CAD build for the part. Positions are in the model's coordinates, mm. A direction names the side the tool comes from. Give positions to 0.01 mm unless a question says otherwise; leave off trailing zeros. Order: outer loops, then holes, each group sorted by start corner. A loop starts at its lowest first (then second) coordinate and runs counter-clockwise, first axis right, second up. Notation, with made-up numbers: (-5, 59.25) -> (12, 59.25) arc R17 cw to (12, 91.25) -> close; hole circle Ø4 at (11, 73.25). An arc over 180 degrees is marked (long way). Answer as CSV lines item,"result".
```python
from build123d import *

# Parameters (mm, degrees)
SKETCH_2_OUTSIDE_W  = 26.11
SKETCH_2_OUTSIDE_H  = 26.11
CUT_EXTRUDE_1_DEPTH = 45.3


with BuildPart() as part:
    # Эскиз1 → Повернуть1 (revolve)
    with BuildSketch(Plane.XY, mode=Mode.PRIVATE) as revolve_1_sk:
        Polygon((-5.3, 0), (-5.3, 6.175), (-5.052146997, 7.1), (0, 7.1), (0, 4), (39.2, 4), (40, 3.2), (40, 0), align=None)
    revolve(revolve_1_sk.sketch.rotate(Axis((-1000, 0, 0), (1, 0, 0)), 90), axis=Axis((-1000, 0, 0), (1, 0, 0)))

    # Эскиз2 outside → Вырез-Вытянуть1 (cut)
    with BuildSketch(Plane.ZY.offset(5.3)):
        Rectangle(SKETCH_2_OUTSIDE_W, SKETCH_2_OUTSIDE_H)
        Polygon((0, 7.505553499), (-6.5, 3.75277675), (-6.5, -3.75277675), (0, -7.505553499), (6.5, -3.75277675), (6.5, 3.75277675), align=None, mode=Mode.SUBTRACT)
    extrude(amount=-CUT_EXTRUDE_1_DEPTH, mode=Mode.SUBTRACT)


solid = part.part
```
1) Band-saw the part on C-C, the plane x = 22. Write the cut outline in (y, z).
Data:
outline,"circle Ø8 at (0, 0)"
2) Pin check, flat tips, straight feed: P1, Ø5, axis at x = 27.5, z = 3.5, coming from the -Y side; P2, Ø2, axis at y = -5.5, z = -5, coming from the -X side; P3, Ø3, axis at x = 31.5, y = 5, coming from the -Z side. Stop position of each tip, or through.
Data:
P1,"stops at y = -3.87"
P2,"stops at x = -5.23"
P3,"stops at z = -1.94"
3) Wall check: line 1 along X through (y, z) = (2.5, -5); line 2 along Y through (x, z) = (9.5, 2.5); line 3 along Z through (x, y) = (33, -1). Give the ranges that are in metal, low to high. Write a range as [from, to].
Data:
line 1,"x = [-5.3, 0]"
line 2,"y = [-3.12, 3.12]"
line 3,"z = [-3.87, 3.87]"
4) Band-saw the part on A-A, the plane y = 0. Write the cut outline in (x, z) (3 decimals).
Data:
outline,"(-5.3, -6.175) -> (-5.213, -6.5) -> (0, -6.5) -> (0, -4) -> (39.2, -4) -> (40, -3.2) -> (40, 3.2) -> (39.2, 4) -> (0, 4) -> (0, 6.5) -> (-5.213, 6.5) -> (-5.3, 6.175) -> close"
5) Which spindle directions (+Z, -Z, +X, -X, +Y, -Y) get a long thin tool onto all of the face, cutting with end or side? Do faces 1 (the flat face through (0, 3, -3)), 2 (the cylindrical face through (-2.491, 3.541, -6.154)). Say none if no direction does.
Data:
face 1,"+X"
face 2,"-Z, +X, -X, +Y"
6) Band-saw the part on B-B, the plane z = 0. Write the cut outline in (x, y) (3 decimals), then the cut area to 3 significant figures.
Data:
outline,"(-5.3, -6.175) -> (-5.052, -7.1) -> (0, -7.1) -> (0, -4) -> (39.2, -4) -> (40, -3.2) -> (40, 3.2) -> (39.2, 4) -> (0, 4) -> (0, 7.1) -> (-5.052, 7.1) -> (-5.3, 6.175) -> close"
area,"394 mm2"
